The listing builds one solid part. Answer for the finished solid, in the listing's coordinates (mm). Face numbers are marked on the shaded views. A direction names the side the tool comes from. Give positions to 0.01 mm unless a question says otherwise; leave off trailing zeros. Write each loop counter-clockwise with the first axis right and the second up, starting at its lowest first coordinate (ties: lowest second). Pieces come first, ordered by that corner, then holes. Notation, with made-up numbers: (71, 46.5) -> (98, 46.5) arc R37 ccw to (98, 83.5) -> close; hole circle Ø1 at (21.25, -5). An arc over 180 degrees is marked (long way). One line per question, with ' | ' between items.
from build123d import *

# Parameters (mm, degrees)
SKETCH1_W           = 42
SKETCH1_H           = 42
BOSS_EXTRUDE1_DEPTH = 33
SKETCH2_R           = 2.5
BOSS_EXTRUDE2_DEPTH = 28
FILLET1_R           = 3
SKETCH3_R           = 1.5
CUT_EXTRUDE1_DEPTH  = 4.5
SKETCH4_R           = 11
BOSS_EXTRUDE3_DEPTH = 2


with BuildPart() as part:
    # Sketch1 → Boss-Extrude1 (new body)
    with BuildSketch(Plane(origin=(0, 0, 0), x_dir=(1, 0, 0), z_dir=(0, 1, 0))):
        with Locations((21, 21)):
            Rectangle(SKETCH1_W, SKETCH1_H)
    extrude(amount=BOSS_EXTRUDE1_DEPTH)

    # Sketch2 → Boss-Extrude2 (add)
    with BuildSketch(Plane(origin=(0, 33, 0), x_dir=(1, 0, 0), z_dir=(0, 1, 0))):
        with Locations(Location((21, 21, 0), (0, 0, 90))):
            Circle(SKETCH2_R)
    extrude(amount=BOSS_EXTRUDE2_DEPTH)

    # Fillet1
    fillet1_edges = [part.edges().sort_by_distance(p)[0] for p in [
        (42, 16.5, -42),
        (42, 16.5, 0),
        (0, 16.5, 0),
        (0, 16.5, -42),
    ]]
    fillet(fillet1_edges, radius=FILLET1_R)

    # Sketch3 → Cut-Extrude1 (cut)
    with BuildSketch(Plane(origin=(0, 33, 0), x_dir=(1, 0, 0), z_dir=(0, 1, 0))):
        with Locations(Location((5.5, 36.5, 0), (0, 0, 270))):
            Circle(SKETCH3_R)
        with Locations(Location((5.5, 5.5, 0), (0, 0, 90))):
            Circle(SKETCH3_R)
        with Locations(Location((36.5, 5.5, 0), (0, 0, 270))):
            Circle(SKETCH3_R)
        with Locations(Location((36.5, 36.5, 0), (0, 0, 90))):
            Circle(SKETCH3_R)
    extrude(amount=-CUT_EXTRUDE1_DEPTH, mode=Mode.SUBTRACT)

    # Sketch4 → Boss-Extrude3 (add)
    with BuildSketch(Plane(origin=(0, 33, 0), x_dir=(1, 0, 0), z_dir=(0, 1, 0))):
        with Locations(Location((21, 21, 0), (0, 0, 270))):
            Circle(SKETCH4_R)
    extrude(amount=BOSS_EXTRUDE3_DEPTH)


solid = part.part
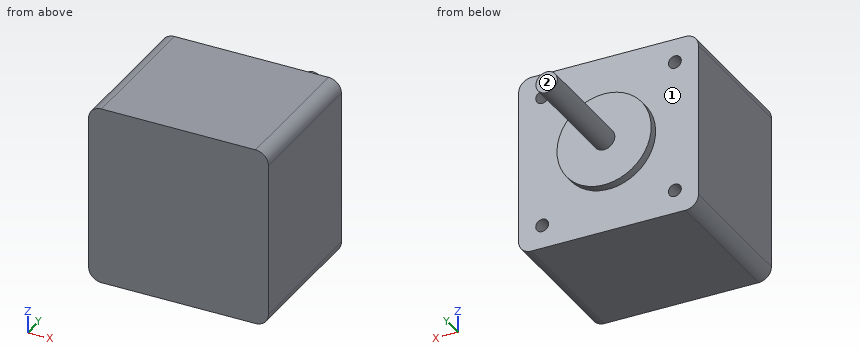
Item 1: Flat-ended cylindrical pins translate along their axes: pin 1 (5 mm diameter, centred on x = 36.5, z = -5.5, fed in from +Y); pin 2 (2.5 mm diameter, centred on x = 5.5, z = -36.5, fed in from +Y); pin 3 (6.5 mm diameter, centred on x = 25.5, z = -26, fed in from +Y). Find the tip coordinate at first contact, or state that the pin passes through.
Answers below:
pin 1: y = 33 | pin 2: y = 28.5 | pin 3: y = 35
Item 2: Consider line 1 (X direction, y = 31.95, z = -5.5); line 2 (X direction, y = 31, z = -5); line 3 (Y direction, x = 9.5, z = -38). Determine where each line is inside the solid, lowest interval first. Write a range as [from, to].
Answers below:
line 1: [0, 4], [7, 35], [38, 42] | line 2: [0, 4.09], [6.91, 35.09], [37.91, 42] | line 3: [0, 33]
Item 3: Find section D-D (x = 16). Write down the section's boundary in (y, z).
Answers below:
outline: (0, -42) -> (33, -42) -> (33, -30.8) -> (35, -30.8) -> (35, -11.2) -> (33, -11.2) -> (33, 0) -> (0, 0) -> close
Item 4: Find section B-B (x = 21). Write down the section's boundary in (y, z), then the cut area to 3 significant figures.
Answers below:
outline: (0, -42) -> (33, -42) -> (33, -32) -> (35, -32) -> (35, -23.5) -> (61, -23.5) -> (61, -18.5) -> (35, -18.5) -> (35, -10) -> (33, -10) -> (33, 0) -> (0, 0) -> close | area: 1,560 mm²
Item 5: A tool of negligible diameter and unlimited length cuts with its end or side. For the marked faces 1 and 2, from which of +Z, -Z, +X, -X, +Y, -Y can it reach the whole face along a straight path? Write none if from no direction.
Answers below:
face 1: +Y | face 2: +Z, -Z, +X, -X, +Y
Item 6: Find section A-A (z = -5.5). Write down the section's boundary in (x, y).
Answers below:
outline: (0, 0) -> (42, 0) -> (42, 33) -> (38, 33) -> (38, 28.5) -> (35, 28.5) -> (35, 33) -> (7, 33) -> (7, 28.5) -> (4, 28.5) -> (4, 33) -> (0, 33) -> close
Item 7: Find section C-C (y = 47.5). Write down the section's boundary in (x, z), then the cut area to 3 significant figures.
Answers below:
outline: circle Ø5 at (21, -21) | area: 19.6 mm²
